Source: CAD feature listing. Evaluate the final solid. Frame: model axes, mm. Face numbers are marked on the shaded views. A direction names the side the tool comes from. Give positions to 0.01 mm unless a question says otherwise; leave off trailing zeros. Loops run counter-clockwise (first coordinate to the right, second up) from the corner with the lowest first, then second, coordinate; pieces in that order, holes last. Notation, with made-up numbers: (-24, -15.5) -> (-1, -15.5) arc R19 ccw to (-1, 15.5) -> close; hole circle Ø7 at (-4.75, 77). An arc over 180 degrees is marked (long way). Put each result on its own line as item: value.
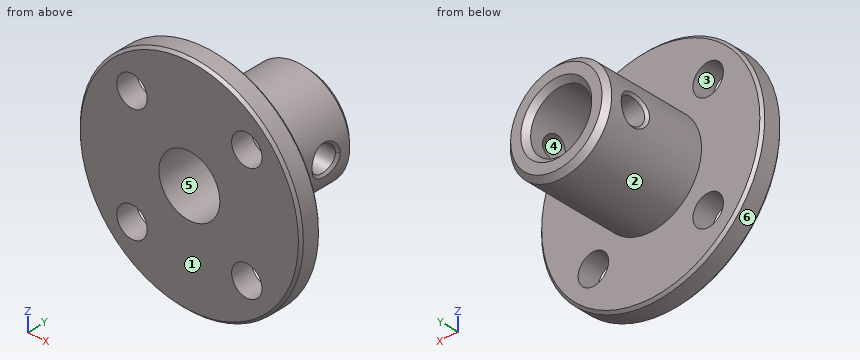
Autodesk Inventor part; units mm, degrees
ref_plane "YZ Plane" through (0, 0, 0) normal (1, 0, 0) x (0, 1, 0)
ref_plane "XZ Plane" through (0, 0, 0) normal (0, 1, 0) x (-1, 0, 0)
ref_plane "XY Plane" through (0, 0, 0) normal (0, 0, 1) x (1, 0, 0)
sketch "Sketch1" plane through (0, 0, 0) normal (0, 0, 1) x (1, 0, 0)
  line L0 (0, 0) -> (11, 0)
  line L1 (11, 0) -> (11, 2.1)
  line L2 (11, 2.1) -> (0, 2.1)
  line L3 (0, 2.1) -> (0, 0)
  line L4 (0, 0) -> (5, 0)
  line L5 (5, 0) -> (5, 12.1)
  line L6 (5, 12.1) -> (0, 12.1)
  line L7 (0, 12.1) -> (0, 0)
  line L8 (0, 12.1) -> (3, 12.1)
  line L9 (3, 12.1) -> (3, 0)
  line L10 (3, 0) -> (0, 0)
  line L11 (0, 0) -> (0, 12.1)
  point P0 (3, 0)
  point P1 (5, 2.1)
  dimension "d0" = 11
  dimension "d1" = 2.1
  dimension "d2" = 5
  dimension "d3" = 12.1
  dimension "d4" = 3
revolve "Revolution1" add sketch "Sketch1" angle 360 about axis through (0, 12.1, 0) along (0, -1, 0) contours L9 L2 L5 L0 | L5 L2 L1 L0 | L9 L6 L5 L2
sketch "Sketch2" plane through (0, 0, 0) normal (0, -1, 0) x (1, 0, 0)
  circle A0 centre (0, 0) radius 8 construction
  line L0 (0, 0) -> (8, 0) construction
  circle A1 centre (8, 0) radius 1.5
  circle A2 centre (5.6569, 5.6569) radius 1.5
  circle A3 centre (0, 8) radius 1.5
  circle A4 centre (-5.6569, 5.6569) radius 1.5
  circle A5 centre (-8, 0) radius 1.5
  circle A6 centre (-5.6569, -5.6569) radius 1.5
  circle A7 centre (0, -8) radius 1.5
  circle A8 centre (5.6569, -5.6569) radius 1.5
  dimension "d6" = 16
  dimension "d7" = 3
  dimension "d10" = 360
extrude "Extrusion1" cut sketch "Sketch2" against normal through all contours A2 | A4 | A6 | A8
sketch "Sketch3" plane through (0, 0, 0) normal (1, 0, 0) x (0, 1, 0)
  line L0 (12.1, 5) -> (12.1, -5)
  line L1 (12.1, 0) -> (0, 0) construction
  circle A0 centre (9.1, 0) radius 1.25
  dimension "d14" = 2.5
  dimension "d15" = 3
extrude "Extrusion2" cut sketch "Sketch3" along normal through all both and the other way through all
chamfer "Chamfer1" distance 0.5 angle 45 2 edges at (-5, 12.1, 0) (-3, 12.1, 0)
chamfer "Chamfer2" distance 0.25 angle 45 5 edges at (-11, 0, 0) (-11, 2.1, 0) (4.8412, 9.0999, -1.25) (4.8412, 9.1, 1.25) (-5, 7.85, -0.0003)
properties part number "Hubs - 6mm" material "Stainless Steel"
(1) Section C-C on z = 6.75. Give the number of separate pieces and of enclosed holes in the cut face, then the cut area to 3 significant figures.
Calculated:
separate pieces: 3
enclosed holes: 0
area: 27.7 mm²
(2) Section A-A on x = 0. Return loops of the section in (y, z).
Calculated:
outline: (0, -10.75) -> (0.25, -11) -> (1.85, -11) -> (2.1, -10.75) -> (2.1, -5) -> (11.6, -5) -> (12.1, -4.5) -> (12.1, -3.5) -> (11.6, -3) -> (0, -3) -> close; (0, 3) -> (11.6, 3) -> (12.1, 3.5) -> (12.1, 4.5) -> (11.6, 5) -> (2.1, 5) -> (2.1, 10.75) -> (1.85, 11) -> (0.25, 11) -> (0, 10.75) -> close
(3) Reachability of the marked faces 1 and 2 from +Z, -Z, +X, -X, +Y, -Y: full face, straight path, thin tool, end or side. Return the list, or none.
Calculated:
face 1: +Z, -Z, +X, -X, -Y
face 2: +Y
(4) Draft query along X for the marked faces 3, 4, 5 and 6. Return one class per face: released by +X, released by -X, zero draft, split by the parting line, or undercut.
Calculated:
face 3: undercut
face 4: zero draft
face 5: undercut
face 6: split by the parting line
(5) Section B-B on y = 4. Return loops of the section in (x, z), then the cut area to 3 significant figures.
Calculated:
outline: circle Ø10 at (0, 0); hole circle Ø6 at (0, 0)
area: 50.3 mm²
(6) Line query: probe 1 along Z at (x, y) = (0, 6); probe 2 along Y at (x, z) = (-10, 2.5); probe 3 along X at (y, z) = (6.25, 2.25). Output: solid intervals per line, ascending. Write a range as from..to.
Calculated:
probe 1: z = -5..-3, 3..5
probe 2: y = 0..2.1
probe 3: x = -4.47..-1.98, 1.98..4.47
(7) First-contact query: P1, Ø5, axis at x = -5.66, z = -5.66, coming from the +Y side; P2, Ø1, axis at y = 10, z = 3, coming from the +X side; P3, Ø4, axis at y = 9.1, z = 0, coming from the +X side. Flat tips, straight axial feed; report the tip coordinate or a pass-through.
Calculated:
P1: stops at y = 2.1
P2: stops at x = 4.33
P3: stops at x = 5
(8) Section D-D on y = 1.5. Return loops of the section in (x, z), then the cut area to 3 significant figures.
Calculated:
outline: circle Ø22 at (0, 0); hole circle Ø3 at (-5.66, -5.66); hole circle Ø3 at (-5.66, 5.66); hole circle Ø6 at (0, 0); hole circle Ø3 at (5.66, -5.66); hole circle Ø3 at (5.66, 5.66)
area: 324 mm²
